```python
from build123d import *

# Parameters (mm, degrees)
BOSS_EXTRUDE1_DEPTH = 31.5
SKETCH2_R           = 2.075
CUT_EXTRUDE1_DEPTH  = 7
CUT_EXTRUDE2_DEPTH  = 10


with BuildPart() as part:
    # Sketch1 → Boss-Extrude1 (new body)
    with BuildSketch(Plane.XY):
        Polygon((0, 0), (0, 12.5), (7.9, 12.5), (7.9, 5.2), (11.3, 5.2), (11.3, 0), align=None)
    extrude(amount=-BOSS_EXTRUDE1_DEPTH)

    # Sketch2 → Cut-Extrude1 (cut)
    with BuildSketch(Plane(origin=(0, 12.5, 0), x_dir=(1, 0, 0), z_dir=(0, 1, 0))):
        with Locations(Location((4, 6, 0), (0, 0, 270))):
            Circle(SKETCH2_R)
        with Locations(Location((4, 25.5, 0), (0, 0, 270))):
            Circle(SKETCH2_R)
    extrude(amount=-CUT_EXTRUDE1_DEPTH, mode=Mode.SUBTRACT)

    # Sketch3 → Cut-Extrude2 (cut)
    with BuildSketch(Plane.XZ):
        Polygon((7.9, -2), (7.9, 0), (11.3, 0), (11.3, -6), align=None)
    extrude(amount=-CUT_EXTRUDE2_DEPTH, mode=Mode.SUBTRACT)


solid = part.part
```
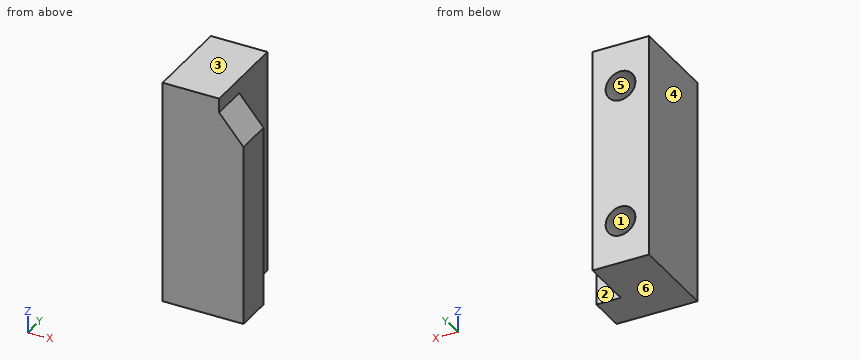
Geometry check sheet. Reference: the model listing, model coordinates, mm. Face numbers are marked on the shaded views. A direction names the side the tool comes from. Coordinates: 2 decimals unless noted, no trailing zeros. Order: outer loops, then holes, each group sorted by start corner. A loop starts at its lowest first (then second) coordinate and runs counter-clockwise, first axis right, second up. Notation, with made-up numbers: (67.25, 9) - (92.25, 9) arc R30 cw to (92.25, 48) - close; hole circle Ø4 at (49, 78.5). An arc over 180 degrees is marked (long way). Answer as a JSON object with one key per item and string values. Group by question number.
Item 1: Scan lines: probe 1 along X at (y, z) = (7.5, -25.5) (3 decimals); probe 2 along Z at (x, y) = (4.75, 9.75); probe 3 along Y at (x, z) = (9.25, -7). Record each from-to range of solid material in increasing order.
Item 2: Draft check along X on the marked faces 4, 5 and 6. Enter one of: +X half, -X half, draft (parallel to the pull), parting line (faces both ways), or undercut.
Item 3: Depth check by flat-ended pin: pin 1 Ø1 at (x, y) = (9, 1.5) entering from +Z; pin 2 Ø2.5 at (x, z) = (10.5, -21.5) entering from +Y. Enter the tip coordinate at first touch or a pass-through.
Item 4: Sectioned sample at B-B, the plane y = 9. Record the cut outline in (x, z) (3 decimals), and give its area (3 significant figures).
Item 5: Sectioned sample at D-D, the plane z = -17. Record the cut outline in (x, y), and give its area (3 significant figures).
Item 6: Tool access check on the marked faces 1, 2 and 3. Record the directions out of +Z, -Z, +X, -X, +Y, -Y that give a thin tool (end or side, any length) a straight path to the whole face; none if there is none.
Item 7: Sectioned sample at A-A, the plane z = -25.5. Record the cut outline in (x, y) (3 decimals), and give its area (3 significant figures).
Item 8: Sectioned sample at C-C, the plane x = 4. Record the cut outline in (y, z) (3 decimals), and give its area (3 significant figures).
Resolved:
{
 "1": {"probe 1": "0 to 1.925, 6.075 to 7.9", "probe 2": "-31.5 to -27.43, -23.57 to -7.93, -4.07 to 0", "probe 3": "0 to 5.2"},
 "2": {"face 4": "-X half", "face 5": "undercut", "face 6": "draft"},
 "3": {"pin 1": "z = -2.71", "pin 2": "y = 5.2"},
 "4": {"outline": "(0, -31.5) - (7.9, -31.5) - (7.9, 0) - (0, 0) - close; hole circle Ø4.15 at (4, -25.5); hole circle Ø4.15 at (4, -6)", "area": "222 mm^2"},
 "5": {"outline": "(0, 0) - (11.3, 0) - (11.3, 5.2) - (7.9, 5.2) - (7.9, 12.5) - (0, 12.5) - close", "area": "116 mm^2"},
 "6": {"face 1": "+Y", "face 2": "+Z, -Z, +X, +Y", "face 3": "+Z, +X, -X, +Y, -Y"},
 "7": {"outline": "(0, 0) - (11.3, 0) - (11.3, 5.2) - (7.9, 5.2) - (7.9, 12.5) - (6.075, 12.5) - (6.075, 5.5) - (1.925, 5.5) - (1.925, 12.5) - (0, 12.5) - close", "area": "87.4 mm^2"},
 "8": {"outline": "(0, -31.5) - (12.5, -31.5) - (12.5, -27.575) - (5.5, -27.575) - (5.5, -23.425) - (12.5, -23.425) - (12.5, -8.075) - (5.5, -8.075) - (5.5, -3.925) - (12.5, -3.925) - (12.5, 0) - (0, 0) - close", "area": "336 mm^2"}
}
